```python
from build123d import *

# Parameters (mm, degrees)
SKETCH_2_W               = 25
SKETCH_2_H               = 2
EXTRUDE_1_DEPTH          = 15
EXTRUDE_1_2_DEPTH        = 15
EXTRUDE_2_DEPTH          = 2.6
EXTRUDE_3_DEPTH          = 15.7
EXTRUDE_4_DEPTH          = 1
EXTRUDE_5_DEPTH          = 2
SKETCH_7_W               = 2
SKETCH_7_H               = 56.3
EXTRUDE_6_DEPTH          = 3.9
SKETCH_8_W               = 4
SKETCH_8_H               = 4
SKETCH_8_R               = 1.2
EXTRUDE_7_DEPTH          = 2
EXTRUDE_START            = -16.35
EXTRUDE_8_DEPTH          = 16.35
CUT_EXTRUDE_1_DEPTH      = 2.6
EXTRUDE_9_DEPTH          = 41.05
SKETCH_12_W              = 10.1
SKETCH_12_H              = 3.07
EXTRUDE_10_DEPTH         = 10
CUT_EXTRUDE_2_DEPTH      = 135.796311397
CUT_EXTRUDE_2_DEPTH_BACK = 135.796311397
EXTRUDE_11_DEPTH         = 3.8
SKETCH_15_W              = 8.65
SKETCH_15_H              = 2
CUT_EXTRUDE_3_DEPTH      = 1.8
CUT_EXTRUDE_4_DEPTH      = 2.4
EXTRUDE_12_DEPTH         = 16.399999999
EXTRUDE_13_REACH         = 109.72
EXTRUDE_14_REACH         = 109.72
CHAMFER_1_SIZE           = 2
CHAMFER_3_SIZE           = 1.8
SKETCH_20_W              = 4
SKETCH_20_H              = 42.789151816
CUT_EXTRUDE_5_DEPTH      = 10
SKETCH_21_W              = 15.7
SKETCH_21_H              = 10
CUT_EXTRUDE_6_DEPTH      = 10


with BuildPart() as part:
    # Sketch 2 → Extrude 1 (new body)
    with BuildSketch(Plane.XY):
        with Locations((-91.85, 1)):
            Rectangle(SKETCH_2_W, SKETCH_2_H)
    extrude(amount=EXTRUDE_1_DEPTH)



with BuildPart() as body_2:
    # Sketch 2 → Extrude 1 2 (new body)
    with BuildSketch(Plane.XY):
        with Locations((-91.85, 59.3)):
            Rectangle(SKETCH_2_W, SKETCH_2_H)
    extrude(amount=EXTRUDE_1_2_DEPTH)


with BuildPart() as part_1:
    add(part.part)

    add(body_2.part)  # Extrude 2 merges body 2
    # Sketch 3 → Extrude 2 (add)
    with BuildSketch(Plane.XY.offset(15)):
        Polygon((-95.7, 2), (-104.35, 2), (-104.35, 0), (-79.35, 0), (-79.35, 60.3), (-104.35, 60.3), (-104.35, 58.3), (-95.7, 58.3), align=None)
    extrude(amount=EXTRUDE_2_DEPTH)

    # Sketch 4 → Extrude 3 (add)
    with BuildSketch(Plane.XY.offset(19.6)):
        Polygon((-104.35, 2), (-104.580416833, 2), (-115.895945033, 11.107600771), (-115.895945033, 49.153887402), (-104.35, 57.869625998), (-104.35, 58.3), (-104.35, 60.2), (-104.416493669, 60.2), (-117.795945033, 50.10019437), (-117.795945033, 10.197880039), (-105.250067231, 0.1), (-104.35, 0.1), align=None)
    extrude(amount=-EXTRUDE_3_DEPTH)

    # Sketch 5 → Extrude 4 (add)
    with BuildSketch(Plane(origin=(0, 0, 3.9), x_dir=(-1, 0, 0), z_dir=(0, 0, -1))):
        Polygon((104.35, 2), (104.35, 57.869625998), (115.895945033, 49.153887402), (115.895945033, 11.107600771), (104.580416833, 2), align=None)
    extrude(amount=-EXTRUDE_4_DEPTH)

    # Sketch 6 → Extrude 5 (add)
    with BuildSketch(Plane(origin=(-104.35, 0, 0), x_dir=(0, 0, -1), z_dir=(1, 0, 0))):
        Polygon((-4.9, 58.3), (-4.9, 57.869625998), (-4.9, 2), (-3.9, 2), (-3.9, 58.3), align=None)
    extrude(amount=EXTRUDE_5_DEPTH)

    # Sketch 7 → Extrude 6 (add)
    with BuildSketch(Plane(origin=(0, 0, 3.9), x_dir=(-1, 0, 0), z_dir=(0, 0, -1))):
        with Locations((103.35, 30.15)):
            Rectangle(SKETCH_7_W, SKETCH_7_H)
    extrude(amount=EXTRUDE_6_DEPTH)

    # Sketch 8 → Extrude 7 (add)
    # profile 1 of 2: a face of its own
    with BuildSketch(Plane(origin=(0, 0, 0), x_dir=(-1, 0, 0), z_dir=(0, 0, -1))):
        with Locations((100.35, 56.3)):
            Rectangle(SKETCH_8_W, SKETCH_8_H)
        with Locations((100.35, 56.3)):
            Circle(SKETCH_8_R, mode=Mode.SUBTRACT)
    # profile 2 of 2: a face of its own
    with BuildSketch(Plane(origin=(0, 0, 0), x_dir=(-1, 0, 0), z_dir=(0, 0, -1))):
        with Locations((100.35, 4)):
            Rectangle(SKETCH_8_W, SKETCH_8_H)
        with Locations((100.35, 4)):
            Circle(SKETCH_8_R, mode=Mode.SUBTRACT)
    extrude(amount=-EXTRUDE_7_DEPTH)

    # Sketch 9 → Extrude 8 (add)
    with BuildSketch(Plane(origin=(-79.35, 0, 0), x_dir=(0, 0, -1), z_dir=(1, 0, 0)).offset(EXTRUDE_START)):
        Polygon((-17.6, 0), (-17.6, -0.5), (0.5, -0.5), (0.5, 0), (0, 0), align=None)
        Polygon((-17.6, 60.8), (-17.6, 60.3), (0, 60.3), (0.5, 60.3), (0.5, 60.8), align=None)
    extrude(amount=EXTRUDE_8_DEPTH)

    # Sketch 10 → Cut-Extrude 1 (cut)
    with BuildSketch(Plane.XY.offset(17.6)):
        Polygon((-95.7, 58.3), (-89.7, 53.15), (-89.7, 7.15), (-95.7, 2), align=None)
    extrude(amount=-CUT_EXTRUDE_1_DEPTH, mode=Mode.SUBTRACT)

    # Sketch 11 → Extrude 9 (add)
    with BuildSketch(Plane(origin=(-79.35, 0, 0), x_dir=(0, 0, -1), z_dir=(1, 0, 0))):
        Polygon((-17.6, 0.1), (0, 0), (0, 2), (-15, 2), (-15, 58.3), (0, 58.3), (0, 60.3), (-17.6, 60.3), align=None)
    extrude(amount=EXTRUDE_9_DEPTH)

    # Sketch 12 → Extrude 10 (add)
    with BuildSketch(Plane(origin=(-38.3, 0, 0), x_dir=(0, 0, -1), z_dir=(1, 0, 0))):
        Polygon((-7.5, 0.042613636), (-7.5, 2), (-15, 2), (-17.6, 2), (-17.6, 0.1), align=None)
        Polygon((-7.5, -4.23), (-7.5, 0.042613636), (-17.6, 0.1), (-17.6, -4.23), align=None)
        with Locations((-12.55, 61.835)):
            Rectangle(SKETCH_12_W, SKETCH_12_H)
        Polygon((-15, 58.3), (-7.5, 58.3), (-7.5, 60.3), (-17.6, 60.3), (-17.6, 58.3), align=None)
    extrude(amount=EXTRUDE_10_DEPTH)

    # Sketch 13 → Cut-Extrude 2 (cut, two sides: drawn at the far end of the back side and taken through both)
    with BuildSketch(Plane.XZ.offset(-58.3).offset(-CUT_EXTRUDE_2_DEPTH_BACK)):
        with BuildLine():
            ThreePointArc((-32.1, 12.55), (-32.838023478, 13.657509681), (-34.144296155, 13.402739117))
            Line((-34.144296155, 13.402739117), (-32.455703844, 11.697260883))
            ThreePointArc((-32.455703844, 11.697260883), (-32.192490319, 12.088023478), (-32.1, 12.55))
        make_face()
        with BuildLine():
            Line((-32.455703844, 11.697260883), (-34.144296155, 13.402739117))
            ThreePointArc((-34.144296155, 13.402739117), (-34.152739117, 11.705703844), (-32.455703844, 11.697260883))
        make_face()
    extrude(amount=CUT_EXTRUDE_2_DEPTH + CUT_EXTRUDE_2_DEPTH_BACK, mode=Mode.SUBTRACT)

    # Sketch 14 → Extrude 11 (add)
    with BuildSketch(Plane.XY.offset(17.6)):
        Polygon((-79.35, 0.1), (-38.42, 0.1), (-38.42, 2), (-38.42, 58.3), (-38.42, 60.3), (-79.35, 60.3), (-79.35, 60.8), (-95.7, 60.8), (-95.7, 60.3), (-104.35, 60.3), (-104.35, 60.2), (-104.35, 58.3), (-95.7, 58.3), (-89.7, 53.15), (-89.7, 7.15), (-95.7, 2), (-104.35, 2), (-104.35, 0.1), (-104.35, 0), (-95.7, 0), (-95.7, -0.5), (-79.35, -0.5), align=None)
    extrude(amount=EXTRUDE_11_DEPTH)

    # Sketch 15 → Cut-Extrude 3 (cut)
    with BuildSketch(Plane.XY.offset(21.4)):
        with Locations((-100.025, 59.3)):
            Rectangle(SKETCH_15_W, SKETCH_15_H)
        with Locations((-100.025, 1)):
            Rectangle(SKETCH_15_W, SKETCH_15_H)
    extrude(amount=-CUT_EXTRUDE_3_DEPTH, mode=Mode.SUBTRACT)

    # Sketch 16 → Cut-Extrude 4 (cut)
    with BuildSketch(Plane(origin=(0, 0, 15), x_dir=(-1, 0, 0), z_dir=(0, 0, -1))):
        Polygon((89.7, 53.15), (95.7, 58.3), (38.3, 58.3), (38.3, 2), (95.7, 2), (89.7, 7.15), align=None)
    extrude(amount=-CUT_EXTRUDE_4_DEPTH, mode=Mode.SUBTRACT)

    # Sketch 17 → Extrude 12 (add)
    with BuildSketch(Plane.XY.offset(21.4)):
        Polygon((-38.42, 60.3), (-38.3, 60.3), (-38.3, 69.47), (-79.35, 60.8), (-79.35, 60.3), align=None)
        Polygon((-79.35, -0.5), (-38.3, -10.33), (-38.3, 0.1), (-38.42, 0.1), (-79.35, 0.1), align=None)
    extrude(amount=-EXTRUDE_12_DEPTH)

    # Extrude 13: up to this plane
    extrude_13_end = Plane(origin=(-15.681436973, 74.247172751, -37.354307927), z_dir=(0.20664708387422698, -0.9784155470587527, 0))
    # Sketch 18 → Extrude 13 (add, up to the surface)
    with BuildSketch(Plane(origin=(-38.3, 0, 0), x_dir=(0, 0, -1), z_dir=(1, 0, 0)), mode=Mode.PRIVATE) as extrude_13_sk1:
        Polygon((-5.000000001, 60.3), (0, 60.3), (-5, 62.15), align=None)
    extrude_13_tool1 = split(extrude(extrude_13_sk1.sketch, amount=-EXTRUDE_13_REACH, mode=Mode.PRIVATE), bisect_by=extrude_13_end, keep=Keep.BOTH, mode=Mode.PRIVATE)
    add(extrude_13_tool1.solids().sort_by_distance((-38.3, 60.916667, 3.333333))[0])

    # Extrude 14: up to this plane
    extrude_14_end = Plane(origin=(-4.416638762, -18.443847527, -37.354307927), z_dir=(-0.23288011181129656, -0.9725054516673715, 0))
    # Sketch 19 → Extrude 14 (add, up to the surface)
    with BuildSketch(Plane(origin=(-38.3, 0, 0), x_dir=(0, 0, -1), z_dir=(1, 0, 0)), mode=Mode.PRIVATE) as extrude_14_sk1:
        Polygon((-5, -1.85), (0, 0), (-5, 0.028409091), align=None)
    extrude_14_tool1 = split(extrude(extrude_14_sk1.sketch, amount=-EXTRUDE_14_REACH, mode=Mode.PRIVATE), bisect_by=extrude_14_end, keep=Keep.BOTH, mode=Mode.PRIVATE)
    add(extrude_14_tool1.solids().sort_by_distance((-38.3, -0.607197, 3.333333))[0])

    # Chamfer 1
    chamfer_1_edges = [part_1.edges().sort_by_distance(p)[0] for p in [
        (-55.629065744, 65.81, 5.000000001),
        (-56.006205493, -6.09, 5.000000001),
    ]]
    chamfer(chamfer_1_edges, length=CHAMFER_1_SIZE)

    # Chamfer 3
    chamfer_3_edges = [part_1.edges().sort_by_distance(p)[0] for p in [
        (-95.7, 59.55, 21.4),
        (-95.7, 0.75, 21.4),
    ]]
    chamfer(chamfer_3_edges, length=CHAMFER_3_SIZE - 0.0001)  # a hair under: the kernel refuses the full size

    # Sketch 20 → Cut-Extrude 5 (cut)
    with BuildSketch(Plane.XY.offset(4.9)):
        Polygon((-106.35, 8.559002447), (-106.35, 51.348154263), (-111.895945033, 47.161662205), (-111.895945033, 13.022802313), align=None)
        with Locations((-104.35, 29.953578355)):
            Rectangle(SKETCH_20_W, SKETCH_20_H)
    extrude(amount=-CUT_EXTRUDE_5_DEPTH, mode=Mode.SUBTRACT)

    # Sketch 21 → Cut-Extrude 6 (cut)
    with BuildSketch(Plane.ZY.offset(117.795945033)):
        with Locations((11.75, 30.149037204)):
            Rectangle(SKETCH_21_W, SKETCH_21_H)
    extrude(amount=-CUT_EXTRUDE_6_DEPTH, mode=Mode.SUBTRACT)


solid = part_1.part
```
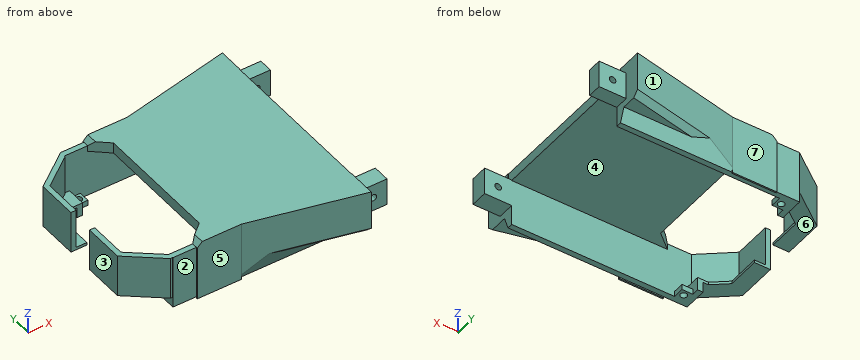
For this review, take the finished solid that the model builds, in its own axes (mm). Face numbers are marked on the shaded views. A direction names the side the tool comes from. Give positions to 0.01 mm unless a question says otherwise; leave off trailing zeros. Write each loop counter-clockwise with the first axis right and the second up, starting at its lowest first coordinate (ties: lowest second). Pieces come first, ordered by that corner, then holes. Notation, with made-up numbers: M 8,86.25 L 32,86.25 A9 ccw 32,92.25 Z; hole C 81.5,26 d7. An arc over 180 degrees is marked long. Answer as a JSON object with one key per item and string values. Group by question number.
Item 1: For probe 1 along Y at (x, z) = (-100.35, 0.6); probe 2 along Y at (x, z) = (-101, 4.25); probe 3 along Z at (x, y) = (-83, 13), list the stretches that pass through material, from the lowest coordinate up. Write a range as [from, to].
Item 2: Draft analysis for pull direction Y (two halves, no side actions). For the marked faces 1, 2, 3 and 4, state which applies: +Y half, -Y half, draft (parallel to the pull), parting line (faces both ways), or undercut.
Item 3: Consider section B-B on x = -100.35. Write out the cut boundary in (y, z), plus the area to 3 significant figures.
Item 4: Tool access review of the marked faces 5, 6 and 7: name each direction out of +Z, -Z, +X, -X, +Y, -Y from which nothing blocks a thin tool from reaching the whole face with its end or side.
Item 5: Consider section C-C on x = -87.5. Write out the cut boundary in (y, z), plus the area to 3 significant figures.
Item 6: Consider section D-D on x = -51.5. Write out the cut boundary in (y, z), plus the area to 3 significant figures.
Item 7: For pin 1 Ø2.5 at (y, z) = (6.5, 2.5) entering from +X; pin 2 Ø10 at (x, z) = (-97, 18.5) entering from +Y; pin 3 Ø10 at (x, z) = (-75.5, 13) entering from +Y, all flat-tipped, find the tip position at first contact; note any pin that passes through.
Item 8: Consider section A-A on y = 38.5. Write out the cut boundary in (x, z).
Check result:
{
 "1": {"probe 1": "y = [0, 2.8], [5.2, 6], [54.3, 55.1], [57.5, 60.3]", "probe 2": "y = [0, 2], [58.3, 60.3]", "probe 3": "z = [17.4, 21.4]"},
 "2": {"face 1": "+Y half", "face 2": "-Y half", "face 3": "draft", "face 4": "undercut"},
 "3": {"outline": "M 0,0 L 2.8,0 L 2.8,2 L 2,2 L 2,19.6 L 0,19.6 Z; M 5.2,0 L 6,0 L 6,2 L 5.2,2 Z; M 54.3,0 L 55.1,0 L 55.1,2 L 54.3,2 Z; M 57.5,0 L 60.3,0 L 60.3,19.6 L 58.3,19.6 L 58.3,2 L 57.5,2 Z", "area": "84.8 mm^2"},
 "4": {"face 5": "+Z, -Z, -X, -Y", "face 6": "-Z, -X, +Y, -Y", "face 7": "+Z, -Z, -X, +Y"},
 "5": {"outline": "M -0.5,-0.5 L 0,-0.5 L 0,0 L 2,0 L 2,17.4 L 58.3,17.4 L 58.3,0 L 60.3,0 L 60.3,-0.5 L 60.8,-0.5 L 60.8,21.4 L -0.5,21.4 Z", "area": "333 mm^2"},
 "6": {"outline": "M -7.17,7 L -5.11,5 L -1.85,5 L 0,0 L 2,0 L 2,17.4 L 58.3,17.4 L 58.3,0 L 60.3,0 L 62.15,5 L 64.64,5 L 66.68,7 L 66.68,21.4 L -7.17,21.4 Z", "area": "538 mm^2"},
 "7": {"pin 1": "stops at x = -98.35", "pin 2": "stops at y = 60.8", "pin 3": "stops at y = 62.67"},
 "8": {"outline": "M -117.8,3.9 L -111.9,3.9 L -111.9,4.9 L -115.9,4.9 L -115.9,19.6 L -117.8,19.6 Z; M -89.7,17.4 L -38.3,17.4 L -38.3,17.6 L -38.42,17.6 L -38.42,21.4 L -89.7,21.4 Z"}
}
